Autodesk Inventor part; units mm, degrees
ref_plane "YZ Plane" through (0, 0, 0) normal (1, 0, 0) x (0, 1, 0)
ref_plane "XZ Plane" through (0, 0, 0) normal (0, 1, 0) x (-1, 0, 0)
ref_plane "XY Plane" through (0, 0, 0) normal (0, 0, 1) x (1, 0, 0)
sketch "Sketch1" plane through (0, 0, 0) normal (0, 1, 0) x (-1, 0, 0)
  line L0 (177, 77.5) -> (-78, 77.5)
  line L1 (-78, 77.5) -> (-78, -77.5)
  line L2 (-78, -77.5) -> (177, -77.5)
  line L3 (177, -77.5) -> (177, 77.5)
  point P0 (0, 0)
  dimension "d0" = 155
  dimension "d1" = 77.5
  dimension "d2" = 78
  dimension "d3" = 255
extrude "Extrusion1" add sketch "Sketch1" along normal blind 8
fillet "Fillet1" radius 15 2 edges at (78, 4, -77.5) (78, 4, 77.5)
sketch "Sketch2" plane through (0, 8, 0) normal (0, 1, 0) x (1, 0, 0)
  arc A0 (63, -77.5) -> (78, -62.5) centre (63, -62.5) ccw
  line L0 (63, -62.5) -> (-62, -62.5)
  line L1 (-62, -62.5) -> (-62, 62.5)
  line L2 (-62, 62.5) -> (63, 62.5)
  line L3 (63, 62.5) -> (63, -62.5)
  point P0 (0, 0)
  dimension "d7" = 125
hole "Hole1" at (-62, 8, 62.5) at (63, 8, 62.5) at (63, 8, -62.5) at (-62, 8, -62.5) direction (0, -1, 0) diameter 10 end through all
sketch "Sketch3" plane through (0, 8, 0) normal (0, 1, 0) x (1, 0, 0)
  circle A0 centre (0, 0) radius 40
  dimension "d15" = 80
extrude "Extrusion2" cut sketch "Sketch3" against normal through all
properties part number "BRACKET BASE"
Read the model definition and answer for the solid it produces. Units are mm, in the model's axes. Round coordinates to 2 decimals unless told otherwise and drop trailing zeros. Write each loop counter-clockwise with the first axis right and the second up, starting at its lowest first coordinate (ties: lowest second). Pieces come first, ordered by that corner, then holes. Notation, with made-up numbers: M -8.75,8 L 4.25,8 A9 cw 4.25,23 Z; hole C -27,68 d7. An arc over 180 degrees is marked long. Use a Markdown table: item, result.
1) Straight lines are drawn through the part: line 1 along Z through (x, y) = (-62, 4); line 2 along X through (y, z) = (3, -62.5); line 3 along X through (y, z) = (1, 61.5). For each, find the intervals that lie inside material, in ascending order. Write a range as [from, to].
Answers follow:
| item | result |
|---|---|
| line 1 | z = [-77.5, -67.5], [-57.5, 57.5], [67.5, 77.5] |
| line 2 | x = [-177, -67], [-57, 58], [68, 78] |
| line 3 | x = [-177, -66.9], [-57.1, 58.1], [67.9, 78] |
2) The part is cut by section B-B (x = 0). Write down the section's boundary in (y, z), plus the area to 3 significant figures.
Answers follow:
| item | result |
|---|---|
| outline | M 0,-77.5 L 8,-77.5 L 8,-40 L 0,-40 Z; M 0,40 L 8,40 L 8,77.5 L 0,77.5 Z |
| area | 600 mm2 |
3) For a pull along Z with two mould halves and no side action, classify faces 1 (the cylindrical face through (58.043, 3.944, 61.849)), 2 (the flat face through (-177, 4, -1)), 3 (the cylindrical face through (73.49, 4.06, 73.22)) as pulls with the +Z half, pulls with the -Z half, needs draft (parallel to the pull), parting line crosses it, or undercut.
Answers follow:
| item | result |
|---|---|
| face 1 | undercut |
| face 2 | needs draft |
| face 3 | pulls with the +Z half |
4) The part is cut by section D-D (y = 3.25). Write down the section's boundary in (x, z), plus the area to 3 significant figures.
Answers follow:
| item | result |
|---|---|
| outline | M -177,-77.5 L 63,-77.5 A15 ccw 78,-62.5 L 78,62.5 A15 ccw 63,77.5 L -177,77.5 Z; hole C -62,-62.5 d10; hole C -62,62.5 d10; hole C 0,0 d80; hole C 63,-62.5 d10; hole C 63,62.5 d10 |
| area | 34,100 mm2 |
5) A flat-ended cylindrical pin translates along its axis: pin 1 (8 mm diameter, centred on x = -62, z = 62.5, fed in from -Y). Find the tip coordinate at first contact, or state that the pin passes through.
Answers follow:
| item | result |
|---|---|
| pin 1 | passes through |
6) The part is cut by section A-A (x = -62). Write down the section's boundary in (y, z), plus the area to 3 significant figures.
Answers follow:
| item | result |
|---|---|
| outline | M 0,-77.5 L 8,-77.5 L 8,-67.5 L 0,-67.5 Z; M 0,-57.5 L 8,-57.5 L 8,57.5 L 0,57.5 Z; M 0,67.5 L 8,67.5 L 8,77.5 L 0,77.5 Z |
| area | 1,080 mm2 |
7) The part is cut by section C-C (z = 0). Write down the section's boundary in (x, y), plus the area to 3 significant figures.
Answers follow:
| item | result |
|---|---|
| outline | M -177,0 L -40,0 L -40,8 L -177,8 Z; M 40,0 L 78,0 L 78,8 L 40,8 Z |
| area | 1,400 mm2 |
